Design review of the part built by this model. Coordinates are the model's own, in mm. Face numbers are marked on the shaded views. A direction names the side the tool comes from. Coordinates: 2 decimals unless noted, no trailing zeros. Loops run counter-clockwise (first coordinate to the right, second up) from the corner with the lowest first, then second, coordinate; pieces in that order, holes last. Notation, with made-up numbers: (69, -23) - (114, -23) arc R27 ccw to (114, 8) - close; hole circle Ø11 at (-28.75, 76.5). An arc over 180 degrees is marked (long way). Answer in a Markdown table with one row per item. Add a question column.
(1) We need section C-C, the plane y = -12.5. Write out the cut boundary in (x, z), plus the area to 3 significant figures.
(2) We need section D-D, the plane z = 5.5. Write out the cut boundary in (x, y), plus the area to 3 significant figures.
(3) Clearance check with flat-ended pins moving along their axes: pin 1 (1.5 mm diameter, centred on x = 0, z = 8, fed in from +Y); pin 2 (3 mm diameter, centred on x = -9.5, y = 0.5, fed in from +Z); pin 3 (5 mm diameter, centred on x = -0.5, y = 4.5, fed in from +Z). State where each tip first meets the part, or that it passes through.
(4) We need section A-A, the plane z = 1.5. Write out the cut boundary in (x, y).
(5) To check wall thickness, follow L1, parallel to Y at x = -17, z = 4.2; L2, parallel to Y at x = 5, z = 0.75; L3, parallel to Y at x = -16, z = 1.5. State the ranges of each line that lie inside material, in increasing order. Write a range as [from, to].
(6) The part is to be moulded in two halves that separate along X. For the marked faces 6, 7, 8 and 9, say which applies: released by +X, released by -X, zero draft, split by the parting line, or undercut.
(7) We need section B-B, the plane x = -17. Write out the cut boundary in (y, z), plus the area to 3 significant figures.
(8) For the marked faces 1, 2, 3, 4 and 5, list the 3-axis set-ups (+Z, -Z, +X, -X, +Y, -Y) from which the entire face can be reached by the end or side of a thin tool; tool diameter is ignored.
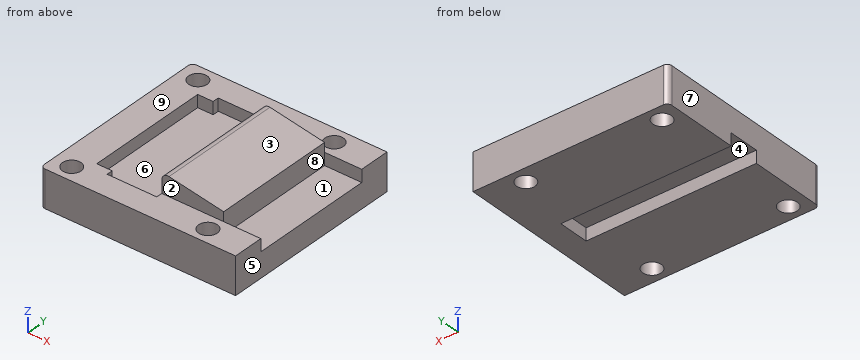
from build123d import *

# Parameters (mm, degrees)
SKETCH1_W                = 30
SKETCH1_H                = 20
BASE_PLATE_DEPTH         = 1
SIDE_WALLS_DEPTH         = 6
SKETCH3_W                = 10
SKETCH3_H                = 20
SWITCH_BLOCK_DEPTH       = 6.5
SKETCH11_W               = 10.5
SKETCH11_H               = 20
SKETCH11_W_2             = 9.5
THICKER_BODY_DEPTH       = 3
SWITCH_BLOCK_ANGLE_DEPTH = 20
SKETCH4_R                = 1.5
M2_SCREWS_DEPTH          = 6
FILLET1_R                = 1
FILLET2_R                = 0.5
FILLET3_R                = 0.5
FILLET4_R                = 0.75
FILLET5_R                = 0.75
SKETCH19_W               = 8
SKETCH19_H               = 22
SPACE_FOR_LEAVER_DEPTH   = 2
SKETCH20_W               = 27.5
SKETCH20_H               = 5
CUT_EXTRUDE1_DEPTH       = 2
CUT_EXTRUDE2_DEPTH       = 26.506893306
CUT_EXTRUDE2_DEPTH_BACK  = 26.506893306
SKETCH21_W               = 20.782145583
SKETCH21_H               = 41.62772639


with BuildPart() as part:
    # Sketch1 → Base Plate (new body)
    with BuildSketch(Plane.XY):
        Rectangle(SKETCH1_W, SKETCH1_H)
    extrude(amount=BASE_PLATE_DEPTH)

    # Sketch2 → Side Walls (add)
    with BuildSketch(Plane(origin=(0, 0, 0), x_dir=(1, 0, 0), z_dir=(0, 0, -1))):
        Polygon((15, 10), (-15, 10), (-15, -10), (15, -10), (15, -15), (-20, -15), (-20, 15), (15, 15), align=None)
    extrude(amount=-SIDE_WALLS_DEPTH)

    # Sketch3 → Switch Block (add)
    with BuildSketch(Plane.XY.offset(1)):
        with Locations((0.5, 0)):
            Rectangle(SKETCH3_W, SKETCH3_H)
    extrude(amount=SWITCH_BLOCK_DEPTH)

    # Sketch11 → Thicker Body (add)
    with BuildSketch(Plane.XY.offset(1)):
        with Locations((-9.75, 0)):
            Rectangle(SKETCH11_W, SKETCH11_H)
        with Locations((10.25, 0)):
            Rectangle(SKETCH11_W_2, SKETCH11_H)
    extrude(amount=THICKER_BODY_DEPTH)

    # Sketch5 → Switch Block Angle (add)
    with BuildSketch(Plane(origin=(0, 10, 0), x_dir=(-1, 0, 0), z_dir=(0, 1, 0))):
        Polygon((4.5, 7.5), (4.5, 9.25), (-5.5, 7.5), align=None)
    extrude(amount=-SWITCH_BLOCK_ANGLE_DEPTH)

    # Sketch4 → M2 Screws (cut)
    with BuildSketch(Plane.XY.offset(6)):
        with Locations((-17, -12.5)):
            Circle(SKETCH4_R)
        with Locations((5, -12.5)):
            Circle(SKETCH4_R)
        with Locations((5, 12.5)):
            Circle(SKETCH4_R)
        with Locations((-17, 12.5)):
            Circle(SKETCH4_R)
    extrude(amount=-M2_SCREWS_DEPTH, mode=Mode.SUBTRACT)

    # Fillet1
    fillet1_edges = [part.edges().sort_by_distance(p)[0] for p in [
        (-4.5, 0, 9.25),
    ]]
    fillet(fillet1_edges, radius=FILLET1_R)

    # Fillet2
    fillet2_edges = [part.edges().sort_by_distance(p)[0] for p in [
        (15, -15, 3),
    ]]
    fillet(fillet2_edges, radius=FILLET2_R)

    # Fillet3
    fillet3_edges = [part.edges().sort_by_distance(p)[0] for p in [
        (15, 15, 3),
    ]]
    fillet(fillet3_edges, radius=FILLET3_R)

    # Fillet4
    fillet4_edges = [part.edges().sort_by_distance(p)[0] for p in [
        (-20, 15, 3),
    ]]
    fillet(fillet4_edges, radius=FILLET4_R)

    # Fillet5
    fillet5_edges = [part.edges().sort_by_distance(p)[0] for p in [
        (-20, -15, 3),
    ]]
    fillet(fillet5_edges, radius=FILLET5_R)

    # Sketch19 → Space for LEaver (cut)
    with BuildSketch(Plane.XY.offset(6)):
        with Locations((-8.5, 0)):
            Rectangle(SKETCH19_W, SKETCH19_H)
    extrude(amount=-SPACE_FOR_LEAVER_DEPTH, mode=Mode.SUBTRACT)

    # Sketch20 → Cut-Extrude1 (cut)
    with BuildSketch(Plane(origin=(0, 0, 0), x_dir=(1, 0, 0), z_dir=(0, 0, -1))):
        with Locations((-6.25, 0)):
            Rectangle(SKETCH20_W, SKETCH20_H)
    extrude(amount=-CUT_EXTRUDE1_DEPTH, mode=Mode.SUBTRACT)

    # Sketch21 → Cut-Extrude2 (cut, two sides: drawn at the far end of the back side and taken through both)
    with BuildSketch(Plane.XY.offset(4).offset(-CUT_EXTRUDE2_DEPTH_BACK)):
        with Locations((21.891072792, -1.973183351)):
            Rectangle(SKETCH21_W, SKETCH21_H)
    extrude(amount=CUT_EXTRUDE2_DEPTH + CUT_EXTRUDE2_DEPTH_BACK, mode=Mode.SUBTRACT)


solid = part.part
Responses:
| question | item | result |
|---|---|---|
| 1 | outline | (-20, 0) - (-18.5, 0) - (-18.5, 6) - (-20, 6) - close; (-15.5, 0) - (3.5, 0) - (3.5, 6) - (-15.5, 6) - close; (6.5, 0) - (11.5, 0) - (11.5, 6) - (6.5, 6) - close |
| 1 | area | 153 mm2 |
| 2 | outline | (-20, -14.25) arc R0.75 ccw to (-19.25, -15) - (11.5, -15) - (11.5, -10) - (5.5, -10) - (5.5, 10) - (11.5, 10) - (11.5, 15) - (-19.25, 15) arc R0.75 ccw to (-20, 14.25) - close; hole circle Ø3 at (-17, -12.5); hole circle Ø3 at (-17, 12.5); hole (-15, -10) - (-12.5, -10) - (-12.5, -11) - (-4.5, -11) - (-4.5, 11) - (-12.5, 11) - (-12.5, 10) - (-15, 10) - close; hole circle Ø3 at (5, -12.5); hole circle Ø3 at (5, 12.5) |
| 2 | area | 570 mm2 |
| 3 | pin 1 | stops at y = 10 |
| 3 | pin 2 | stops at z = 4 |
| 3 | pin 3 | stops at z = 8.99 |
| 4 | outline | (-20, -14.25) arc R0.75 ccw to (-19.25, -15) - (11.5, -15) - (11.5, 15) - (-19.25, 15) arc R0.75 ccw to (-20, 14.25) - (-20, 2.5) - (7.5, 2.5) - (7.5, -2.5) - (-20, -2.5) - close; hole circle Ø3 at (-17, -12.5); hole circle Ø3 at (-17, 12.5); hole circle Ø3 at (5, -12.5); hole circle Ø3 at (5, 12.5) |
| 5 | L1 | y = [-15, -14], [-11, 11], [14, 15] |
| 5 | L2 | y = [-15, -14], [-11, -2.5], [2.5, 11], [14, 15] |
| 5 | L3 | y = [-15, -13.62], [-11.38, -2.5], [2.5, 11.38], [13.62, 15] |
| 6 | face 6 | undercut |
| 6 | face 7 | released by -X |
| 6 | face 8 | released by +X |
| 6 | face 9 | zero draft |
| 7 | outline | (-15, 0) - (-14, 0) - (-14, 6) - (-15, 6) - close; (-11, 0) - (-2.5, 0) - (-2.5, 2) - (2.5, 2) - (2.5, 0) - (11, 0) - (11, 6) - (-11, 6) - close; (14, 0) - (15, 0) - (15, 6) - (14, 6) - close |
| 7 | area | 134 mm2 |
| 8 | face 1 | +Z, +X |
| 8 | face 2 | +Z, +X, -X, -Y |
| 8 | face 3 | +Z, +X, +Y, -Y |
| 8 | face 4 | -Z, -X |
| 8 | face 5 | +Z, -Z, +X, +Y, -Y |
